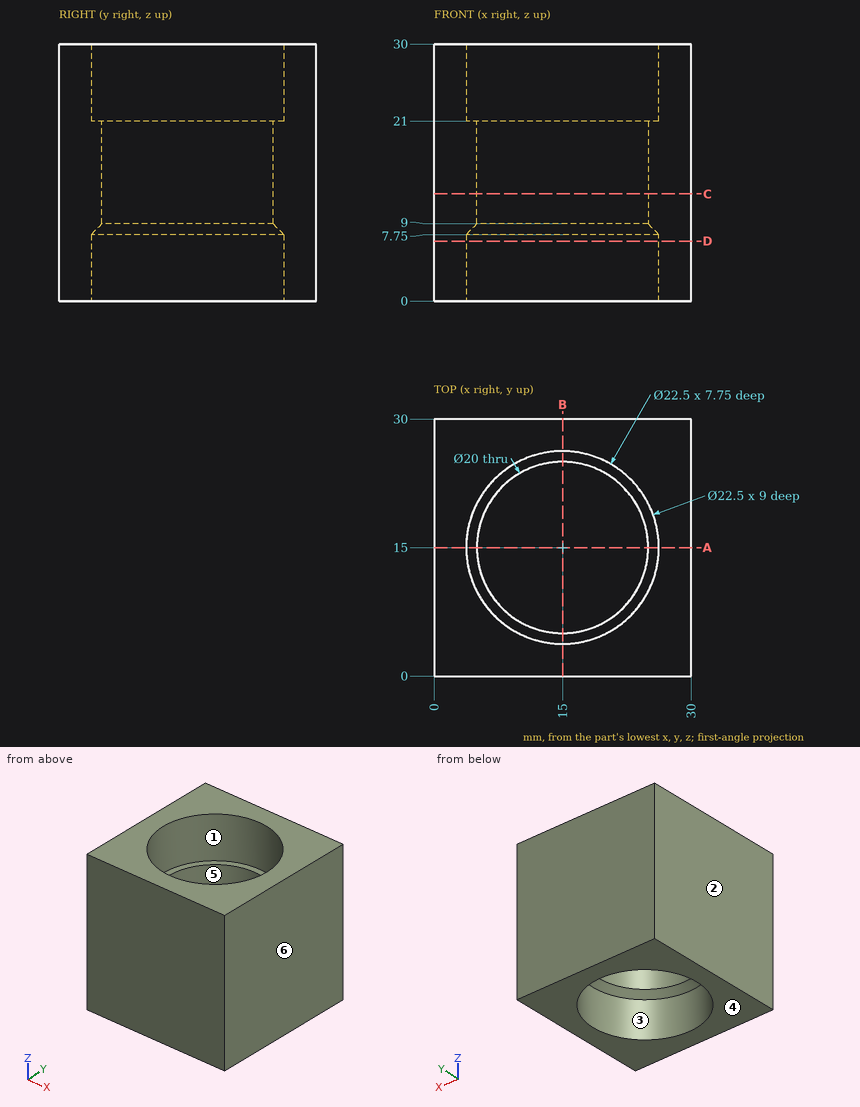
For this review, use the dimensioned drawing (mm, ordinates from the lowest corner) and the shaded views. A direction names the side the tool comes from. Round coordinates to 2 decimals unless told otherwise and drop trailing zeros. Write each loop counter-clockwise with the first axis right and the second up, starting at its lowest first coordinate (ties: lowest second). Pieces come first, ordered by that corner, then holes. Notation, with made-up numbers: (86.5, 44.5) -> (122.5, 44.5) arc R25 cw to (122.5, 59.5) -> close; hole circle Ø1 at (8, -24). An arc over 180 degrees is marked (long way). One line per item, written item: value. Start each with the question number.
Q1. Add section D-D (z = 7). Give the boundary of the cut face in (x, y), then the cut area to 3 significant figures.
Q2. Add section A-A (y = 15). Give the boundary of the cut face in (x, z).
Q3. The part is to be moulded in two halves that separate along X. For the marked faces 4, 5 and 6, say which applies: pulls with the +X half, pulls with the -X half, needs draft (parallel to the pull), parting line crosses it, or undercut.
Q4. Insertion check: P1, Ø3, axis at x = 15, y = 6, coming from the +Z side. The pin has a flat end and moves straight along its axis. Give the tip position at first contact, or say it passes through.
Q5. To check wall thickness, follow probe 1 along Y at (x, z) = (15, 17.25); probe 2 along Y at (x, z) = (15, 26). State the ranges of each line that lie inside material, in increasing order.
Q6. Tool access review of the marked faces 1, 2 and 3: name each direction out of +Z, -Z, +X, -X, +Y, -Y from which nothing blocks a thin tool from reaching the whole face with its end or side.
Q7. Add section C-C (z = 12.5). Give the boundary of the cut face in (x, y), then the cut area to 3 significant figures.
Response:
1. outline: (0, 0) -> (30, 0) -> (30, 30) -> (0, 30) -> close; hole circle Ø22.5 at (15, 15)
1. area: 502 mm^2
2. outline: (0, 0) -> (3.75, 0) -> (3.75, 7.75) -> (5, 9) -> (5, 21) -> (3.75, 21) -> (3.75, 30) -> (0, 30) -> close; (25, 9) -> (26.25, 7.75) -> (26.25, 0) -> (30, 0) -> (30, 30) -> (26.25, 30) -> (26.25, 21) -> (25, 21) -> close
3. face 4: needs draft
3. face 5: undercut
3. face 6: pulls with the +X half
4. P1: stops at z = 21
5. probe 1: y = 0 to 5, 25 to 30
5. probe 2: y = 0 to 3.75, 26.25 to 30
6. face 1: +Z
6. face 2: +Z, -Z, -X, +Y, -Y
6. face 3: -Z
7. outline: (0, 0) -> (30, 0) -> (30, 30) -> (0, 30) -> close; hole circle Ø20 at (15, 15)
7. area: 586 mm^2
